from build123d import *

# Parameters (mm, degrees)
REVOLVE1_ANGLE = 180


with BuildPart() as part:
    # Sketch1 → Revolve1 (revolve)
    with BuildSketch(Plane.XY):
        with BuildLine():
            Line((-203.2, 46.355), (-203.2, 41.4909))
            Line((-203.2, 41.4909), (-199.161210988, 41.4909))
            ThreePointArc((-199.161210988, 41.4909), (-196.989383077, 41.873851858), (-195.079509666, 42.976517786))
            Line((-195.079509666, 42.976517786), (-186.641312326, 50.057006062))
            ThreePointArc((-186.641312326, 50.057006062), (-185.604253506, 50.765114497), (-184.448126603, 51.255297255))
            ThreePointArc((-184.448126603, 51.255297255), (-98.994308497, 71.366370982), (-11.557, 79.210311199))
            ThreePointArc((-11.557, 79.210311199), (-7.739510449, 78.92004648), (-4.044584679, 77.917547785))
            ThreePointArc((-4.044584679, 77.917547785), (-1.493258292, 77.212550225), (1.143, 76.975))
            Line((1.143, 76.975), (8.763, 76.975))
            Line((8.763, 76.975), (8.763, 79.375))
            Line((8.763, 79.375), (1.143, 79.375))
            Line((1.143, 79.375), (0, 80.518))
            ThreePointArc((0, 80.518), (-103.025907626, 71.917734953), (-203.2, 46.355))
        make_face()
    revolve(axis=Axis((0, 0, 0), (-1, 0, 0)), revolution_arc=REVOLVE1_ANGLE)


solid = part.part
Geometry: final body of the model. Coordinates: model frame, mm. A direction names the side the tool comes from. Give positions to 0.01 mm unless a question says otherwise; leave off trailing zeros. Put each result on its own line as item: value. Start each with the question number.
1) Ray query, line 1 along Y through (x, z) = (-120, -41.5); line 2 along Y through (x, z) = (-169, -20); line 3 along Z through (x, y) = (-15, 50.5). Return the intervals inside material, ascending.
2) Pull-direction query (Y, two-part tool) for faces 4 (the cylindrical face through (-201.15, 0.91, -41.48)), 5 (the flat face through (-106, 71, 0)), 6 (the conical face through (0.9, 1.7, -79.6)), 7 (the conical face through (-194.55, 0.95, -43.41)); classes: pulls with the +Y half, pulls with the -Y half, needs draft (parallel to the pull), parting line crosses it, or undercut.
3) Access query for faces 1 (the flat face through (-203.2, -4, -42)), 2 (the cylindrical face through (5.006, 1.693, -76.956)), 3 (the cylindrical face through (4.9, 1.745, -79.356)). Directions: +Z, -Z, +X, -X, +Y, -Y. A direction counts if a zero-diameter tool reaches every point of the face in a straight line with its end or side. Return the directions, or none.
4) Contact query for flat-ended pins moving along their axis: pin 1 (6 mm diameter, centred on x = -58, y = 53, fed in from +Z); pin 2 (1 mm diameter, centred on x = -159.5, y = 22, fed in from -Z); pin 3 (4 mm diameter, centred on x = -86.5, z = -45, fed in from -Y). Output: stop coordinate, or through.
Verdict:
1. line 1: -54.9 to -53.36, 53.36 to 54.9
1. line 2: -53.48 to -52.14, 52.14 to 53.48
1. line 3: -62.48 to -60.93
2. face 4: undercut
2. face 5: needs draft
2. face 6: parting line crosses it
2. face 7: undercut
3. face 1: +Z, -Z, -X, +Y, -Y
3. face 2: +Z, +X
3. face 3: -Z, +X
4. pin 1: z = -52.24
4. pin 2: z = -55.74
4. pin 3: y = -60.84
